Autodesk Inventor part; units mm, degrees
ref_plane "YZ Plane" through (0, 0, 0) normal (1, 0, 0) x (0, 1, 0)
ref_plane "XZ Plane" through (0, 0, 0) normal (0, 1, 0) x (-1, 0, 0)
ref_plane "XY Plane" through (0, 0, 0) normal (0, 0, 1) x (1, 0, 0)
sketch "Sketch1" plane through (0, 0, 0) normal (0, 0, 1) x (1, 0, 0)
  line L0 (-21.7703, 20.0792) -> (29.0297, 20.0792)
  line L1 (29.0297, 20.0792) -> (29.0297, -5.3208)
  line L2 (29.0297, -5.3208) -> (-21.7703, -5.3208)
  line L3 (-21.7703, -5.3208) -> (-21.7703, 20.0792)
  dimension "d0" = 25.4
  dimension "d1" = 50.8
extrude "Extrusion1" add sketch "Sketch1" along normal blind 436.88
shell "Shell1" thickness 3.175 removed faces 2 at (-4.8369, 11.6125, 436.88) at (-4.8369, 11.6125, 0)
draft "FaceDraft1" angle 8.3 pull direction (0, -1, 0) faces at (-3.7786, 19.0209, 0) fixed edges at (3.6297, 20.0792, 0)
properties part number "FE-00013-05"
The listing builds one solid part. Answer for the finished solid, in the listing's coordinates (mm). A direction names the side the tool comes from. Coordinates: 2 decimals unless noted, no trailing zeros. Order: outer loops, then holes, each group sorted by start corner. A loop starts at its lowest first (then second) coordinate and runs counter-clockwise, first axis right, second up. Notation, with made-up numbers: (49, -27.75) -> (107, -27.75) arc R24 cw to (107, 2.25) -> close; hole circle Ø7 at (14.25, 9). An arc over 180 degrees is marked (long way). Answer in a Markdown table with one row per item. Add a question column.
Item 1: Which of the six approach directions +Z, -Z, +X, -X, +Y, -Y give full straight-line access (tool end or side, diameter ignored) to faces 1 (the face through (3, 20.079, 215)), 2 (the face through (-18.595, 7, 216))?
Item 2: Find section B-B (y = 7). Write down the section's boundary in (x, z), then the cut area to 3 significant figures.
Item 3: Find section A-A (x = 7). Write down the section's boundary in (y, z).
Item 4: Find section C-C (z = 279). Write down the section's boundary in (x, y), then the cut area to 3 significant figures.
Item 5: Find the intervals of material crossed by L1, parallel to X at y = 1.5, z = 42; L2, parallel to Y at x = -17.5, z = 64.5; L3, parallel to Z at x = -19, y = 17, in increasing order. Write a range as from..to.
Result set:
| question | item | result |
|---|---|---|
| 1 | face 1 | +Z, -Z, +X, -X, +Y |
| 1 | face 2 | +Z, -Z |
| 2 | outline | (-21.77, 1.91) -> (-18.6, 1.91) -> (-18.6, 436.88) -> (-21.77, 436.88) -> close; (25.85, 1.91) -> (29.03, 1.91) -> (29.03, 436.88) -> (25.85, 436.88) -> close |
| 2 | area | 2,760 mm² |
| 3 | outline | (-5.32, 3.71) -> (-2.15, 3.24) -> (-2.15, 436.88) -> (-5.32, 436.88) -> close; (16.9, 0.46) -> (20.08, 0) -> (20.08, 436.88) -> (16.9, 436.88) -> close |
| 4 | outline | (-21.77, -5.32) -> (29.03, -5.32) -> (29.03, 20.08) -> (-21.77, 20.08) -> close; hole (-18.6, -2.15) -> (25.85, -2.15) -> (25.85, 16.9) -> (-18.6, 16.9) -> close |
| 4 | area | 444 mm² |
| 5 | L1 | x = -21.77..-18.6, 25.85..29.03 |
| 5 | L2 | y = -5.32..-2.15, 16.9..20.08 |
| 5 | L3 | z = 0.45..436.88 |
